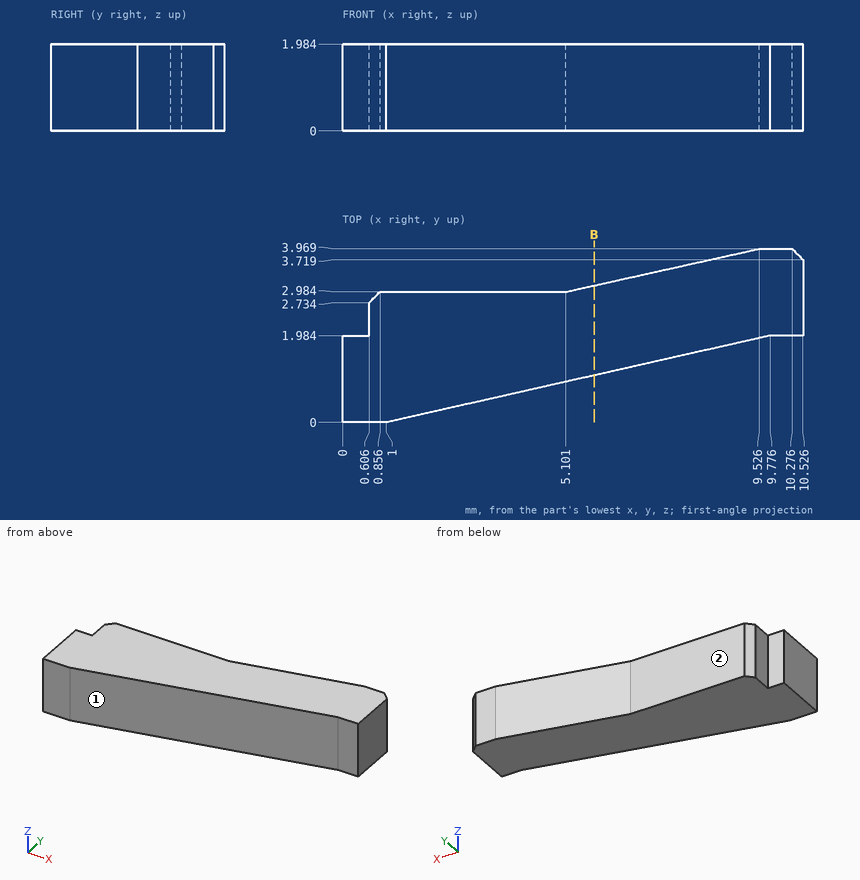
Geometry: see drawing. Coordinates: mm, zero at the bounding-box minimum. A direction names the side the tool comes from. Round coordinates to 2 decimals unless told otherwise and drop trailing zeros. Loops run counter-clockwise (first coordinate to the right, second up) from the corner with the lowest first, then second, coordinate; pieces in that order, holes last.
(1) Section query B-B (x = 5.75). Output: boundary loops of the cut face in (y, z) (1 decimal).
From the geometry:
outline: (1.1, 0) - (3.1, 0) - (3.1, 2) - (1.1, 2) - close
(2) Contact query for flat-ended pins moving along their axis: pin 1 Ø0.6 at (y, z) = (2.5, 0.5) entering from -X; pin 2 Ø0.8 at (x, z) = (10, 1) entering from -Y (1 decimal); pin 3 Ø0.6 at (x, z) = (4, 1) entering from +Y. Output: stop coordinate, or through.
From the geometry:
pin 1: stops at x = 0.61
pin 2: stops at y = 1.9
pin 3: stops at y = 2.98
(3) Material intervals for probe 1 along X at (y, z) = (2.1, 1.55); probe 2 along Y at (x, z) = (1, 0.25) (1 decimal); probe 3 along Y at (x, z) = (7.5, 0.2), sorted ascending.
From the geometry:
probe 1: x = 0.61 to 10.53
probe 2: y = 0 to 3
probe 3: y = 1.47 to 3.52
(4) Access query for the marked faces 1 and 2. Directions: +Z, -Z, +X, -X, +Y, -Y. A direction counts if a zero-diameter tool reaches every point of the face in a straight line with its end or side. Return the directions, or none.
From the geometry:
face 1: +Z, -Z, +X, -Y
face 2: +Z, -Z, -X, +Y
